Source: CAD feature listing. Evaluate the final solid. Frame: model axes, mm. A direction names the side the tool comes from. Give positions to 0.01 mm unless a question says otherwise; leave off trailing zeros. Write item = value, one per line.
from build123d import *

# Parameters (mm, degrees)
SKETCH1_W               = 100
SKETCH1_H               = 80
SKETCH1_R               = 1
BOSS_EXTRUDE1_DEPTH     = 5
SKETCH2_R               = 2
CUT_EXTRUDE1_DEPTH      = 1
CUT_EXTRUDE1_DEPTH_BACK = 2.5
SKETCH3_R               = 1
CUT_EXTRUDE2_DEPTH      = 6
SKETCH5_R               = 1.5
CUT_EXTRUDE4_DEPTH      = 2.5


with BuildPart() as part:
    # Sketch1 → Boss-Extrude1 (new body)
    with BuildSketch(Plane(origin=(0, 0, 0), x_dir=(1, 0, 0), z_dir=(0, 1, 0))):
        with Locations((50, 40)):
            Rectangle(SKETCH1_W, SKETCH1_H)
        with Locations((95, 75)):
            Circle(SKETCH1_R, mode=Mode.SUBTRACT)
        with Locations((5, 75)):
            Circle(SKETCH1_R, mode=Mode.SUBTRACT)
        with Locations((5, 5)):
            Circle(SKETCH1_R, mode=Mode.SUBTRACT)
        with Locations((95, 5)):
            Circle(SKETCH1_R, mode=Mode.SUBTRACT)
        with Locations((95, 65)):
            Circle(SKETCH1_R, mode=Mode.SUBTRACT)
        with Locations((95, 15)):
            Circle(SKETCH1_R, mode=Mode.SUBTRACT)
        with Locations((5, 15)):
            Circle(SKETCH1_R, mode=Mode.SUBTRACT)
        with Locations((5, 65)):
            Circle(SKETCH1_R, mode=Mode.SUBTRACT)
    extrude(amount=BOSS_EXTRUDE1_DEPTH)

    # Sketch2 → Cut-Extrude1 (cut, two sides)
    with BuildSketch(Plane(origin=(0, 5, 0), x_dir=(1, 0, 0), z_dir=(0, 1, 0))) as cut_extrude1_sk:
        with Locations((5, 75)):
            Circle(SKETCH2_R)
        with Locations((95, 75)):
            Circle(SKETCH2_R)
        with Locations((95, 5)):
            Circle(SKETCH2_R)
        with Locations((5, 5)):
            Circle(SKETCH2_R)
        with Locations((5, 65)):
            Circle(SKETCH2_R)
        with Locations((95, 65)):
            Circle(SKETCH2_R)
        with Locations((95, 15)):
            Circle(SKETCH2_R)
        with Locations((5, 15)):
            Circle(SKETCH2_R)
    extrude(amount=CUT_EXTRUDE1_DEPTH, mode=Mode.SUBTRACT)
    extrude(cut_extrude1_sk.sketch, amount=-CUT_EXTRUDE1_DEPTH_BACK, mode=Mode.SUBTRACT)

    # Sketch3 → Cut-Extrude2 (cut, through all)
    with BuildSketch(Plane(origin=(0, 5, 0), x_dir=(1, 0, 0), z_dir=(0, 1, 0))):
        with Locations((58.8, 8)):
            Circle(SKETCH3_R)
        with Locations((69.8, 8)):
            Circle(SKETCH3_R)
        with Locations((58.8, 2)):
            Circle(SKETCH3_R)
        with Locations((69.8, 2)):
            Circle(SKETCH3_R)
        with Locations((58.8, 78)):
            Circle(SKETCH3_R)
        with Locations((69.8, 72)):
            Circle(SKETCH3_R)
        with Locations((69.8, 78)):
            Circle(SKETCH3_R)
        with Locations((58.8, 72)):
            Circle(SKETCH3_R)
    extrude(amount=-CUT_EXTRUDE2_DEPTH, mode=Mode.SUBTRACT)

    # Sketch5 → Cut-Extrude4 (cut)
    with BuildSketch(Plane(origin=(0, 5, 0), x_dir=(1, 0, 0), z_dir=(0, 1, 0))):
        with Locations((58.8, 8)):
            Circle(SKETCH5_R)
        with Locations((58.8, 2)):
            Circle(SKETCH5_R)
        with Locations((69.8, 2)):
            Circle(SKETCH5_R)
        with Locations((69.8, 8)):
            Circle(SKETCH5_R)
        with Locations((58.8, 78)):
            Circle(SKETCH5_R)
        with Locations((58.8, 72)):
            Circle(SKETCH5_R)
        with Locations((69.8, 72)):
            Circle(SKETCH5_R)
        with Locations((69.8, 78)):
            Circle(SKETCH5_R)
    extrude(amount=-CUT_EXTRUDE4_DEPTH, mode=Mode.SUBTRACT)


solid = part.part
1. Pull-direction query (Z, two-part tool) for faces 1 (the flat face through (49, 2, 0)), 2 (the cylindrical face through (94.2, 1.2, -64.4)), 3 (the flat face through (100, 2, -39)); classes: +Z half, -Z half, draft (parallel to the pull), parting line (faces both ways), or undercut.
Derived:
face_1 = +Z half
face_2 = undercut
face_3 = draft
2. First-contact query: pin 1 Ø1.5 at (x, y) = (57, 4.5) entering from +Z; pin 2 Ø0.9 at (x, z) = (58.5, -2.5) entering from +Y. Flat tips, straight axial feed; report the tip coordinate or a pass-through.
Derived:
pin_1 = 0
pin_2 = 2.5
3. Reachability of faces 4 (the cylindrical face through (58, 1.3, -77.4)), 5 (the cylindrical face through (70.49, 3.77, -6.67)) from +Z, -Z, +X, -X, +Y, -Y: full face, straight path, thin tool, end or side. Return the list, or none.
Derived:
face_4 = +Y, -Y
face_5 = +Y
4. Cut plane A-A, the plane y = 4.15. Count the separate pieces of the cut face and the enclosed holes in it, then the cut area to 3 significant figures.
Derived:
separate_pieces = 1
enclosed_holes = 16
area = 7,840 mm²
5. Material intervals for probe 1 along Z at (x, y) = (58.8, 1.7); probe 2 along Z at (x, y) = (69.8, 3.6); probe 3 along X at (y, z) = (3.2, -15), sorted ascending. Write a range as from..to.
Derived:
probe_1 = -80..-79, -77..-73, -71..-9, -7..-3, -1..0
probe_2 = -80..-79.5, -76.5..-73.5, -70.5..-9.5, -6.5..-3.5, -0.5..0
probe_3 = 0..3, 7..93, 97..100
